```python
from build123d import *

# Parameters (mm, degrees)
F0_R     = 125
F1_DEPTH = 250
F1_TAPER = 8
F2_W     = 40
F2_H     = 250
F3_DEPTH = 150
F7_R     = 150
F8_DEPTH = 46.8815590493


with BuildPart() as f1:
    # F0 (on Top) → F1 (new body)
    with BuildSketch(Plane.XY):
        Circle(F0_R)
    extrude(amount=F1_DEPTH, taper=F1_TAPER)

    # F2 (on Right) → F3 (cut)
    with BuildSketch(Plane.YZ):
        with Locations((0, 125)):
            Rectangle(F2_W, F2_H)
    extrude(amount=-F3_DEPTH, mode=Mode.SUBTRACT)

    # F7 (on line) → F8 (cut, through all)
    with BuildSketch(Plane(origin=(-30.3201091399, 0, 215.7387865532), x_dir=(0.9902680687, 0, 0.139173101), z_dir=(0.139173101, 0, -0.9902680687))):
        Circle(F7_R)
    extrude(amount=-F8_DEPTH, mode=Mode.SUBTRACT)


solid = f1.part
```
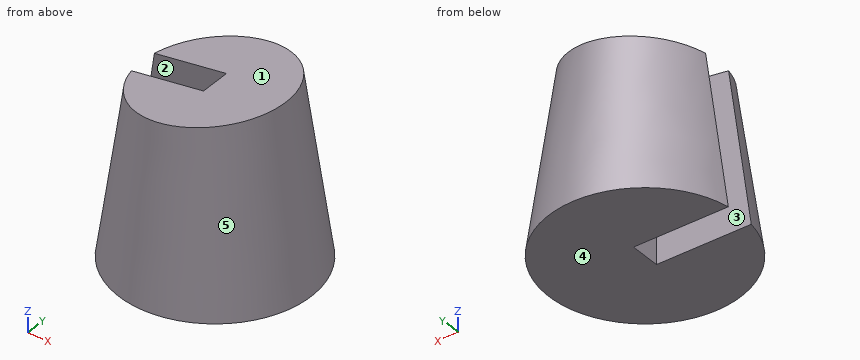
The listing builds one solid part. Answer for the finished solid, in the listing's coordinates (mm). Face numbers are marked on the shaded views. A direction names the side the tool comes from. Give positions to 0.01 mm unless a question says otherwise; leave off trailing zeros. Order: outer loops, then holes, each group sorted by start corner. A loop starts at its lowest first (then second) coordinate and runs counter-clockwise, first axis right, second up. Notation, with made-up numbers: (6.25, 78.25) -> (25.25, 78.25) arc R7 cw to (25.25, 91.25) -> close; hole circle Ø3 at (-37, 35.25). An arc over 180 degrees is marked (long way). Write each question's results on one line, items separated by ' | '.
Q1. Each of these flat-tipped pins is pushed along its axis until it touches: P1, Ø4, axis at y = -26, z = 122.5, coming from the +X side; P2, Ø6, axis at y = 49.5, z = 167, coming from the -X side; P3, Ø1, axis at x = 23.5, z = 53.5, coming from the -Y side. Where does it stop, or does it pass through?
Checked values:
P1: stops at x = 105.16 | P2: stops at x = -90.33 | P3: stops at y = -115.23
Q2. The part is cut by section A-A, the plane y = 0. Give the vertices of the cut face in (x, z).
Checked values:
outline: (0, 0) -> (125, 0) -> (92.26, 232.97) -> (0, 220) -> close
Q3. Which of the six approach directions +Z, -Z, +X, -X, +Y, -Y give full straight-line access (tool end or side, diameter ignored) to the marked faces 1 and 2?
Checked values:
face 1: +Z, -X, +Y, -Y | face 2: +Z, -Z, -X
Q4. The part is cut by section B-B, the plane z = 105. Give the vertices of the cut face in (x, y), and give its area (3 significant figures).
Checked values:
outline: (-108.41, -20) arc R110.24 ccw (long way) to (-108.41, 20) -> (0, 20) -> (0, -20) -> close | area: 33,800 mm^2
Q5. Straight lines are drawn through the part: probe 1 along Y at (x, z) = (-7, 79); probe 2 along Y at (x, z) = (-8.5, 216.5); probe 3 along Z at (x, y) = (82.5, 31.5). For each, find the intervals that lie inside material, in ascending order. Write a range as from..to.
Checked values:
probe 1: y = -113.68..-20, 20..113.68 | probe 2: y = -94.19..-20, 20..94.19 | probe 3: z = 0..231.59
Q6. Determine the mould class of the marked faces 3, 4 and 5 for opening direction Y: pulls with the +Y half, pulls with the -Y half, needs draft (parallel to the pull), parting line crosses it, or undercut.
Checked values:
face 3: undercut | face 4: needs draft | face 5: parting line crosses it
